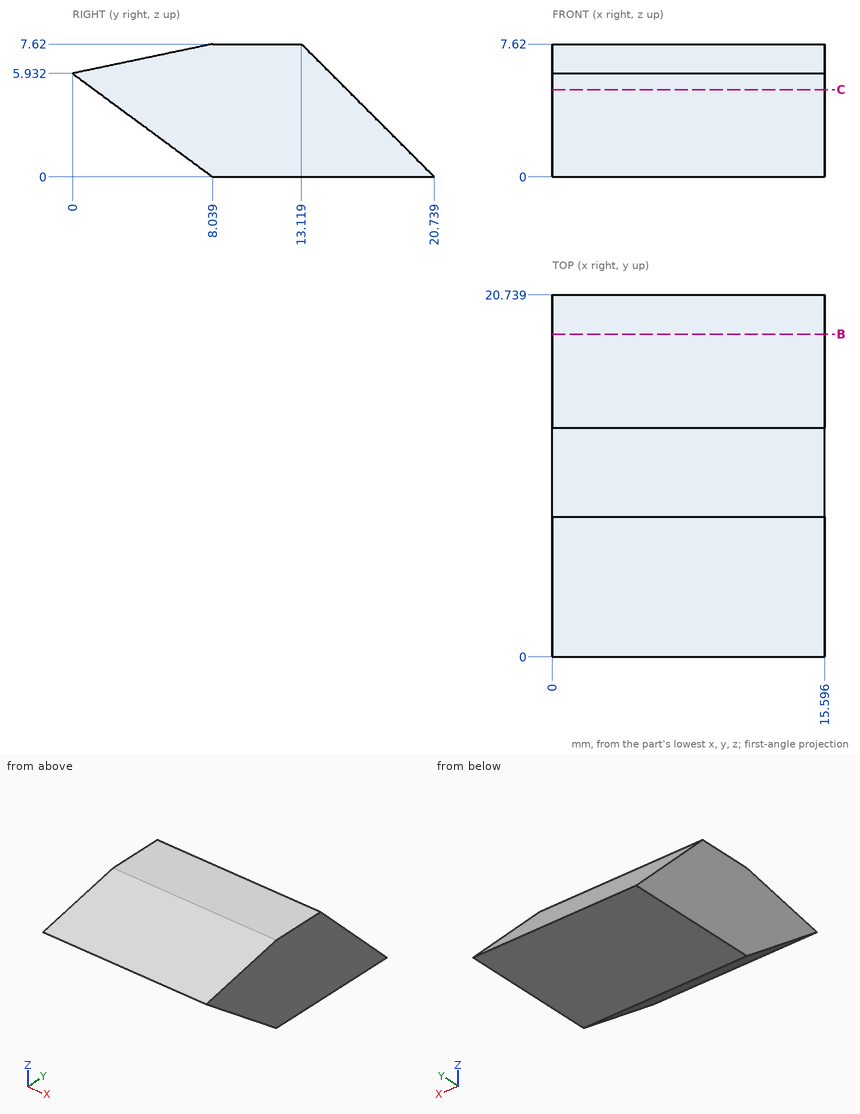
Check sheet for the drawn part. Datum: minimum x, y, z corner. Units: mm. Round coordinates to 2 decimals unless told otherwise and drop trailing zeros. Loops run counter-clockwise (first coordinate to the right, second up) from the corner with the lowest first, then second, coordinate; pieces in that order, holes last. Notation, with made-up numbers: M 38.25,25 L 84.25,25 A23 cw 84.25,37 Z; hole C 11,77.25 d4. An arc over 180 degrees is marked long. Write each question's results on one line, items separated by ' | '.
1) Scan lines: L1, parallel to Y at x = 8.75, z = 4 (1 decimal); L2, parallel to Y at x = 11.25, z = 1.75 (1 decimal); L3, parallel to Z at x = 7.5, y = 7.75 (1 decimal). Record each from-to range of solid material in increasing order. Write a range as from..to.
Checks:
L1: y = 2.6..16.7 | L2: y = 5.7..19 | L3: z = 0.2..7.6
2) Section check B-B on y = 18.5. Record the boundary of the cut face in (x, z) (1 decimal).
Checks:
outline: M 0,0 L 15.6,0 L 15.6,2.2 L 0,2.2 Z
3) Section check C-C on z = 5. Record the boundary of the cut face in (x, y) (1 decimal), then the cut area to 3 significant figures.
Checks:
outline: M 0,1.3 L 15.6,1.3 L 15.6,15.7 L 0,15.7 Z | area: 226 mm2
4) Gauge pin test, flat ends, axial feed: P1, Ø4, axis at x = 6.5, z = 3.5, coming from the +Y side; P2, Ø1, axis at x = 2, y = 6.5, coming from the -Z side; P3, Ø1.5, axis at x = 7, z = 3.5, coming from the +Y side. Record the tip position at first contact, or that the pin passes through.
Checks:
P1: stops at y = 19.24 | P2: stops at z = 0.77 | P3: stops at y = 17.99
